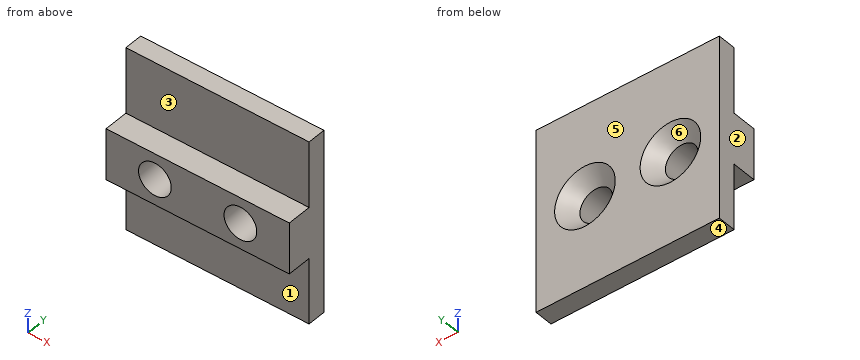
```python
from build123d import *

# Parameters (mm, degrees)
SKETCH1_W                                       = 19.05
SKETCH1_H                                       = 5.334
BOSS_EXTRUDE1_DEPTH                             = 2.54
SKETCH2_W                                       = 19.05
SKETCH2_H                                       = 19.05
BOSS_EXTRUDE2_DEPTH                             = 1.905
CSK_FOR_M3_FLAT_HEAD_MACHINE_SCREW1_D           = 3.4
CSK_FOR_M3_FLAT_HEAD_MACHINE_SCREW1_CSINK_D     = 6.3
CSK_FOR_M3_FLAT_HEAD_MACHINE_SCREW1_CSINK_ANGLE = 90


with BuildPart() as part:
    # Sketch1 → Boss-Extrude1 (new body)
    with BuildSketch(Plane(origin=(0, 0, 0), x_dir=(1, 0, 0), z_dir=(0, 1, 0))):
        Rectangle(SKETCH1_W, SKETCH1_H)
    extrude(amount=BOSS_EXTRUDE1_DEPTH)

    # Sketch2 → Boss-Extrude2 (add)
    with BuildSketch(Plane(origin=(0, 2.54, 0), x_dir=(1, 0, 0), z_dir=(0, 1, 0))):
        Rectangle(SKETCH2_W, SKETCH2_H)
    extrude(amount=BOSS_EXTRUDE2_DEPTH)

    # CSK for M3 Flat Head Machine Screw1 (through all)
    with Locations(Plane(origin=(0, 4.445, 0), x_dir=(1, 0, 0), z_dir=(0, 1, 0))):
        with Locations((-4.445, 0), (4.445, 0)):
            CounterSinkHole(CSK_FOR_M3_FLAT_HEAD_MACHINE_SCREW1_D / 2, CSK_FOR_M3_FLAT_HEAD_MACHINE_SCREW1_CSINK_D / 2, counter_sink_angle=CSK_FOR_M3_FLAT_HEAD_MACHINE_SCREW1_CSINK_ANGLE)


solid = part.part
```
Here's how the part is built. I have some questions about the finished solid (model axes, mm). Face numbers are marked on the shaded views. A direction names the side the tool comes from. Coordinates: 2 decimals unless noted, no trailing zeros. Write each loop counter-clockwise with the first axis right and the second up, starting at its lowest first coordinate (ties: lowest second). Pieces come first, ordered by that corner, then holes. Notation, with made-up numbers: (44.25, 86.5) - (76.25, 86.5) arc R29 cw to (76.25, 118.5) - close; hole circle Ø9 at (3, -18.75). An arc over 180 degrees is marked (long way). One line per item, written item: value.
1) I'm going to push flat-ended pins straight in: P1, Ø2, axis at x = -0.5, z = 7.5, coming from the -Y side; P2, Ø0.8, axis at x = -2.5, y = 1, coming from the -Z side; P3, Ø5.5, axis at x = -4.445, z = 0, coming from the -Y side; P4, Ø0.8, axis at x = 3.5, y = 0.5, coming from the +Z side. Where does each tip first touch, or does it pass through?
Model answer:
P1: stops at y = 2.54
P2: stops at z = -2.67
P3: stops at y = 0
P4: stops at z = 2.67
2) On a 3-axis mill with a long thin cutter (end or side, diameter ignored), from which of +Z, -Z, +X, -X, +Y, -Y can I reach the whole of each face in a straight line? I mean the marked faces 1, 2 and 3. Say none if no direction works.
Model answer:
face 1: -Z, +X, -X, -Y
face 2: +Z, -Z, -X, +Y, -Y
face 3: +Z, +X, -X, -Y
3) Suppose I cut it at C-C on x = 0.25. Write out the boundary of the cut face in (y, z) (3 decimals).
Model answer:
outline: (0, -2.667) - (2.54, -2.667) - (2.54, -9.525) - (4.445, -9.525) - (4.445, 9.525) - (2.54, 9.525) - (2.54, 2.667) - (0, 2.667) - close
4) Suppose I cut it at A-A on z = 0. Write out the boundary of the cut face in (x, y) (3 decimals), and give its area (3 significant figures).
Model answer:
outline: (-9.525, 0) - (-6.145, 0) - (-6.145, 2.995) - (-7.595, 4.445) - (-9.525, 4.445) - close; (-2.745, 0) - (2.745, 0) - (2.745, 2.995) - (1.295, 4.445) - (-1.295, 4.445) - (-2.745, 2.995) - close; (6.145, 0) - (9.525, 0) - (9.525, 4.445) - (7.595, 4.445) - (6.145, 2.995) - close
area: 50.2 mm²
5) I need wall thicknesses on line 1 along Z through (x, y) = (0, 2.15); line 2 along Z through (x, y) = (-4.25, 3.8) (3 decimals); line 3 along Y through (x, z) = (4.25, 4.25) (3 decimals). Which ranges of each line are inside material? Lowest first, please.
Model answer:
line 1: z = -2.67 to 2.67
line 2: z = -9.525 to -2.497, 2.497 to 9.525
line 3: y = 2.54 to 4.445
6) Suppose I cut it at D-D on z = 7. Write out the boundary of the cut face in (x, y) (3 decimals).
Model answer:
outline: (-9.525, 2.54) - (9.525, 2.54) - (9.525, 4.445) - (-9.525, 4.445) - close
7) Suppose I cut it at B-B on y = 0.4. Write out the boundary of the cut face in (x, z) (3 decimals).
Model answer:
outline: (-9.525, -2.667) - (9.525, -2.667) - (9.525, 2.667) - (-9.525, 2.667) - close; hole circle Ø3.4 at (-4.445, 0); hole circle Ø3.4 at (4.445, 0)
8) We'd pull the mould along Z, two halves only. Please class the marked faces 4, 5 and 6: pulls with the +Z half, pulls with the -Z half, needs draft (parallel to the pull), parting line crosses it, or undercut.
Model answer:
face 4: pulls with the -Z half
face 5: needs draft
face 6: undercut
